Model file for the job. Use its own axes, mm. Round coordinates to 2 decimals unless told otherwise and drop trailing zeros. Order: outer loops, then holes, each group sorted by start corner. A loop starts at its lowest first (then second) coordinate and runs counter-clockwise, first axis right, second up. Notation, with made-up numbers: (88, -19) -> (103, -19) arc R14 ccw to (103, -6) -> close; hole circle Ø6 at (6, 77.25). An arc over 180 degrees is marked (long way). Put each result on its own line as item: value. Start each with the question number.
Q1. Cut at C-C, the plane x = 9.5. List the corners of the cut face in (y, z).
Q2. Cut at A-A, the plane x = -11. List the corners of the cut face in (y, z).
Q3. Probe L1, parallel to X at y = 0.9, z = 0; L2, parallel to Z at x = 57, y = 0.3; L3, parallel to X at y = 0.6, z = -128.5. List the from-to ranges inside material, lowest first.
Q4. Cut at B-B, the plane y = 0.3. State how many separate pieces and enclosed holes the cut face has, and give its area (3 significant figures).
Q5. Flat gauge pin, fed straight in: P1, Ø0.8, axis at x = -82.5, y = 1, coming from the -Z side. Where does the tip first touch, or does it go through?
from build123d import *

# Parameters (mm, degrees)
BOSS_EXTRU_1_DEPTH           = 1.5
CHANFREIN1_SIZE              = 30
CHANFREIN1_SIZE2             = 35.752607778
ENL_V_MAT_EXTRU_1_REACH      = 164.257
ESQUISSE2_R                  = 2.5
ESQUISSE2_R_2                = 1.5
ESQUISSE5_R                  = 1.5
ENL_V_MAT_EXTRU_4_DEPTH      = 163.256741
CONG_2_R                     = 6.5
ESQUISSE3_R                  = 1.5
ENL_V_MAT_EXTRU_2_DEPTH      = 163.256741
ENL_V_MAT_EXTRU_3_DEPTH      = 163.256741
ENL_V_MAT_EXTRU_3_DEPTH_BACK = 163.256741
ESQUISSE4_R                  = 8.15
ESQUISSE4_R_2                = 19.5
ESQUISSE4_R_3                = 1.5
ENL_V_MAT_EXTRU_5_REACH      = 164.257
ESQUISSE6_W                  = 3
ESQUISSE6_H                  = 32
ESQUISSE6_R                  = 1.5
CONG_1_R                     = 3


with BuildPart() as part:
    # Esquisse1 → Boss.-Extru.1 (new body)
    with BuildSketch(Plane(origin=(0, 0, 0), x_dir=(1, 0, 0), z_dir=(0, 1, 0))):
        Polygon((-90, 135), (90, 135), (90, 88.309833424), (55, 70), (55, 0), (-90, 0), align=None)
    extrude(amount=BOSS_EXTRU_1_DEPTH)

    # Chanfrein1
    chanfrein1_edges = [part.edges().sort_by_distance(p)[0] for p in [
        (-90, 0.75, -135),
        (90, 0.75, -135),
    ]]
    chanfrein1_side = [part.faces().sort_by_distance(p)[0] for p in [
        (0, 0.75, -135),
    ]]
    chamfer(chanfrein1_edges, length=CHANFREIN1_SIZE, length2=CHANFREIN1_SIZE2, reference=chanfrein1_side[0])

    # Esquisse2 → Enlèv. mat.-Extru.1 (cut, up to next)
    with BuildSketch(Plane(origin=(0, 1.5, 0), x_dir=(1, 0, 0), z_dir=(0, 1, 0)), mode=Mode.PRIVATE) as enl_v_mat_extru_1_sk1:
        with Locations(Location((-50, 90, 0), (0, 0, 270))):
            Circle(ESQUISSE2_R)
    enl_v_mat_extru_1_tool1 = extrude(enl_v_mat_extru_1_sk1.sketch, amount=-ENL_V_MAT_EXTRU_1_REACH, mode=Mode.PRIVATE) & part.part
    # Esquisse2 → Enlèv. mat.-Extru.1 (cut, up to next)
    with BuildSketch(Plane(origin=(0, 1.5, 0), x_dir=(1, 0, 0), z_dir=(0, 1, 0)), mode=Mode.PRIVATE) as enl_v_mat_extru_1_sk2:
        with Locations(Location((50, 90, 0), (0, 0, 270))):
            Circle(ESQUISSE2_R)
    enl_v_mat_extru_1_tool2 = extrude(enl_v_mat_extru_1_sk2.sketch, amount=-ENL_V_MAT_EXTRU_1_REACH, mode=Mode.PRIVATE) & part.part
    # Esquisse2 → Enlèv. mat.-Extru.1 (cut, up to next)
    with BuildSketch(Plane(origin=(0, 1.5, 0), x_dir=(1, 0, 0), z_dir=(0, 1, 0)), mode=Mode.PRIVATE) as enl_v_mat_extru_1_sk3:
        with Locations(Location((50, 40, 0), (0, 0, 270))):
            Circle(ESQUISSE2_R_2)
    enl_v_mat_extru_1_tool3 = extrude(enl_v_mat_extru_1_sk3.sketch, amount=-ENL_V_MAT_EXTRU_1_REACH, mode=Mode.PRIVATE) & part.part
    add(enl_v_mat_extru_1_tool1.solids().sort_by_distance((-50, 1.5, -90))[0], mode=Mode.SUBTRACT)
    add(enl_v_mat_extru_1_tool2.solids().sort_by_distance((50, 1.5, -90))[0], mode=Mode.SUBTRACT)
    add(enl_v_mat_extru_1_tool3.solids().sort_by_distance((50, 1.5, -40))[0], mode=Mode.SUBTRACT)

    # Esquisse5 → Enlèv. mat.-Extru.4 (cut, through all)
    with BuildSketch(Plane(origin=(0, 1.5, 0), x_dir=(1, 0, 0), z_dir=(0, 1, 0))):
        with Locations(Location((85, 93.309833424, 0), (0, 0, 270))):
            Circle(ESQUISSE5_R)
        with Locations(Location((65.087362858, 80.91994096, 0), (0, 0, 270))):
            Circle(ESQUISSE5_R)
        with Locations(Location((-56.969000222, 128.5, 0), (0, 0, 270))):
            Circle(ESQUISSE5_R)
        with Locations(Location((0, 128.5, 0), (0, 0, 270))):
            Circle(ESQUISSE5_R)
        with Locations(Location((56.969000222, 128.5, 0), (0, 0, 270))):
            Circle(ESQUISSE5_R)
    extrude(amount=-ENL_V_MAT_EXTRU_4_DEPTH, mode=Mode.SUBTRACT)

    # Congé2
    cong_2_edges = [part.edges().sort_by_distance(p)[0] for p in [
        (90, 0.75, -88.309833424),
        (-60, 0.75, -135),
        (60, 0.75, -135),
        (90, 0.75, -99.247392222),
        (-90, 0.75, -99.247392222),
    ]]
    fillet(cong_2_edges, radius=CONG_2_R)

    # Symétrie1: part across plane


with BuildPart() as part_1:
    add(part.part)
    add(part.part.mirror(Plane(origin=(55, 1.5, 0), x_dir=(1, 0, 0), z_dir=(0, 0, -1))))

    # Esquisse3 → Enlèv. mat.-Extru.2 (cut, through all)
    with BuildSketch(Plane(origin=(0, 1.5, 0), x_dir=(1, 0, 0), z_dir=(0, 1, 0))):
        with Locations(Location((32.5, -27.5, 0), (0, 0, 270))):
            Circle(ESQUISSE3_R)
        with Locations(Location((32.5, 27.5, 0), (0, 0, 270))):
            Circle(ESQUISSE3_R)
        with Locations(Location((-32.5, -27.5, 0), (0, 0, 90))):
            Circle(ESQUISSE3_R)
        with Locations(Location((-32.5, 27.5, 0), (0, 0, 90))):
            Circle(ESQUISSE3_R)
        with BuildLine():
            Line((42, 4), (55, 4))
            ThreePointArc((55, 4), (59, 0), (55, -4))
            Line((55, -4), (42, -4))
            ThreePointArc((42, -4), (38, 0), (42, 4))
        make_face()
    extrude(amount=-ENL_V_MAT_EXTRU_2_DEPTH, mode=Mode.SUBTRACT)

    # Esquisse4 → Enlèv. mat.-Extru.3 (cut, two sides: drawn at the far end of the back side and taken through both)
    with BuildSketch(Plane(origin=(0, 1.5, 0), x_dir=(1, 0, 0), z_dir=(0, 1, 0)).offset(-ENL_V_MAT_EXTRU_3_DEPTH_BACK)):
        with Locations(Location((-28, -90, 0), (0, 0, 270))):
            Circle(ESQUISSE4_R)
        with Locations(Location((0, 90, 0), (0, 0, 270))):
            Circle(ESQUISSE4_R_2)
        with Locations(Location((16, 106, 0), (0, 0, 270))):
            Circle(ESQUISSE4_R_3)
        with Locations(Location((-16, 106, 0), (0, 0, 270))):
            Circle(ESQUISSE4_R_3)
        with Locations(Location((-16, 74, 0), (0, 0, 270))):
            Circle(ESQUISSE4_R_3)
        with Locations(Location((16, 74, 0), (0, 0, 270))):
            Circle(ESQUISSE4_R_3)
    extrude(amount=ENL_V_MAT_EXTRU_3_DEPTH + ENL_V_MAT_EXTRU_3_DEPTH_BACK, mode=Mode.SUBTRACT)

    # Esquisse6 → Enlèv. mat.-Extru.5 (cut, up to next)
    with BuildSketch(Plane(origin=(0, 1.5, 0), x_dir=(1, 0, 0), z_dir=(0, 1, 0)), mode=Mode.PRIVATE) as enl_v_mat_extru_5_sk1:
        Polygon((-90, 86), (-90, -80), (-80, -80), (-80, -48), (-80, 86), align=None)
    enl_v_mat_extru_5_tool1 = extrude(enl_v_mat_extru_5_sk1.sketch, amount=-ENL_V_MAT_EXTRU_5_REACH, mode=Mode.PRIVATE) & part_1.part
    # Esquisse6 → Enlèv. mat.-Extru.5 (cut, up to next)
    with BuildSketch(Plane(origin=(0, 1.5, 0), x_dir=(1, 0, 0), z_dir=(0, 1, 0)), mode=Mode.PRIVATE) as enl_v_mat_extru_5_sk2:
        with Locations((-78.5, -64)):
            Rectangle(ESQUISSE6_W, ESQUISSE6_H)
    enl_v_mat_extru_5_tool2 = extrude(enl_v_mat_extru_5_sk2.sketch, amount=-ENL_V_MAT_EXTRU_5_REACH, mode=Mode.PRIVATE) & part_1.part
    # Esquisse6 → Enlèv. mat.-Extru.5 (cut, up to next)
    with BuildSketch(Plane(origin=(0, 1.5, 0), x_dir=(1, 0, 0), z_dir=(0, 1, 0)), mode=Mode.PRIVATE) as enl_v_mat_extru_5_sk3:
        with Locations(Location((-69.5, 0, 0), (0, 0, 270))):
            Circle(ESQUISSE6_R)
    enl_v_mat_extru_5_tool3 = extrude(enl_v_mat_extru_5_sk3.sketch, amount=-ENL_V_MAT_EXTRU_5_REACH, mode=Mode.PRIVATE) & part_1.part
    add(enl_v_mat_extru_5_tool1.solids().sort_by_distance((-85, 1.5, -3))[0], mode=Mode.SUBTRACT)
    add(enl_v_mat_extru_5_tool2.solids().sort_by_distance((-78.5, 1.5, 64))[0], mode=Mode.SUBTRACT)
    add(enl_v_mat_extru_5_tool3.solids().sort_by_distance((-69.5, 1.5, 0))[0], mode=Mode.SUBTRACT)

    # Congé1
    cong_1_edges = [part_1.edges().sort_by_distance(p)[0] for p in [
        (-77, 0.75, 80),
        (-77, 0.75, 48),
        (-80, 0.75, -86),
        (-90, 0.75, 80),
        (-90, 0.75, -86),
    ]]
    fillet(cong_1_edges, radius=CONG_1_R - 0.0001)  # a hair under: the kernel refuses the full size


solid = part_1.part
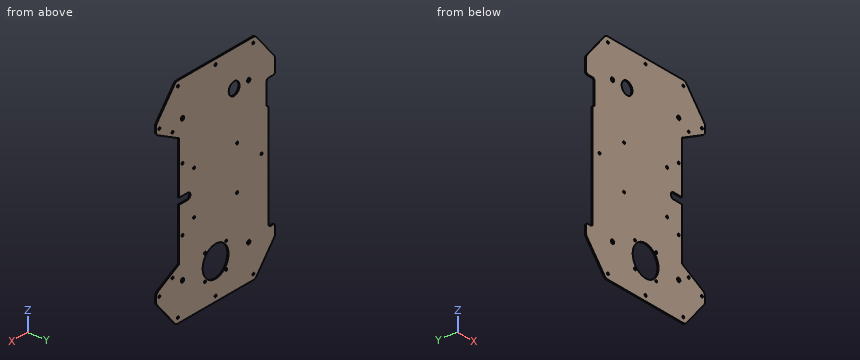
Ans:
1. outline: (0, -135) -> (1.5, -135) -> (1.5, -107.03) -> (0, -107.03) -> close; (0, -72.97) -> (1.5, -72.97) -> (1.5, 135) -> (0, 135) -> close
2. outline: (0, -135) -> (1.5, -135) -> (1.5, -106.1) -> (0, -106.1) -> close; (0, -73.9) -> (1.5, -73.9) -> (1.5, 135) -> (0, 135) -> close
3. L1: x = -80 to -71, -68 to 38
3. L2: z = -135 to -130, -127 to -71.05, 71.05 to 127, 130 to 135
3. L3: x = -65.45 to -58.47, -55.47 to -1.5, 1.5 to 55.47, 58.47 to 65.45
4. separate pieces: 1
4. enclosed holes: 27
4. area: 37,400 mm^2
5. P1: stops at z = -108.66
